from build123d import *

# Parameters (mm, degrees)
SKETCH1_W           = 29.3
SKETCH1_H           = 17
SKETCH1_R           = 1.25
BOSS_EXTRUDE1_DEPTH = 1.15
FILLET1_R           = 2.5
SKETCH2_W           = 6.962283529
SKETCH2_H           = 3.729158124
BOSS_EXTRUDE2_DEPTH = 3.5
SKETCH3_W           = 0.499386372
SKETCH3_H           = 0.1
SKETCH3_W_2         = 0.535571303
SKETCH3_W_3         = 0.69846846
CUT_EXTRUDE1_DEPTH  = 5.5
SKETCH4_W           = 6.01860052
SKETCH4_H           = 2.306780687
CUT_EXTRUDE2_DEPTH  = 3.5
SKETCH5_W           = 5.89277612
SKETCH5_H           = 4.278029639
BOSS_EXTRUDE3_DEPTH = 1
SKETCH6_W           = 3.208522229
SKETCH6_H           = 3.166580762
BOSS_EXTRUDE4_DEPTH = 1
SKETCH7_W           = 6
SKETCH7_H           = 6
BOSS_EXTRUDE5_DEPTH = 3
SKETCH8_W           = 6
SKETCH8_H           = 6
SKETCH8_R           = 1.858011724
SKETCH8_R_2         = 0.603796911
CUT_EXTRUDE3_DEPTH  = 0.5
SKETCH10_R          = 4
BOSS_EXTRUDE6_DEPTH = 10
SKETCH11_R          = 2.5
CUT_EXTRUDE4_DEPTH  = 2
SKETCH12_R          = 2.5
SKETCH12_R_2        = 2.4
CUT_EXTRUDE5_DEPTH  = 2
FILLET2_R           = 2
SKETCH13_R          = 2.5
SKETCH13_R_2        = 2.4
CUT_EXTRUDE6_DEPTH  = 2
FILLET3_R           = 2
CHAMFER1_SIZE       = 0.5
SKETCH14_R          = 3.6
SKETCH14_R_2        = 3.5
CUT_EXTRUDE7_DEPTH  = 2


with BuildPart() as part:
    # Sketch1 → Boss-Extrude1 (new body)
    with BuildSketch(Plane(origin=(0, 0, 0), x_dir=(1, 0, 0), z_dir=(0, 1, 0))):
        Rectangle(SKETCH1_W, SKETCH1_H)
        with Locations(Location((-12.15, 6, 0), (0, 0, 270))):
            Circle(SKETCH1_R, mode=Mode.SUBTRACT)
        with Locations(Location((-12.15, -6, 0), (0, 0, 270))):
            Circle(SKETCH1_R, mode=Mode.SUBTRACT)
        with Locations(Location((12.15, -6, 0), (0, 0, 270))):
            Circle(SKETCH1_R, mode=Mode.SUBTRACT)
        with Locations(Location((12.15, 6, 0), (0, 0, 270))):
            Circle(SKETCH1_R, mode=Mode.SUBTRACT)
    extrude(amount=BOSS_EXTRUDE1_DEPTH)

    # Fillet1
    fillet1_edges = [part.edges().sort_by_distance(p)[0] for p in [
        (14.65, 0.575, 8.5),
        (-14.65, 0.575, 8.5),
        (-14.65, 0.575, -8.5),
        (14.65, 0.575, -8.5),
    ]]
    fillet(fillet1_edges, radius=FILLET1_R)

    # Sketch2 → Boss-Extrude2 (add)
    with BuildSketch(Plane(origin=(0, 1.15, 0), x_dir=(1, 0, 0), z_dir=(0, 1, 0))):
        with Locations((-2.998814894, -6.635420938)):
            Rectangle(SKETCH2_W, SKETCH2_H)
    extrude(amount=BOSS_EXTRUDE2_DEPTH)

    # Sketch3 → Cut-Extrude1 (cut)
    with BuildSketch(Plane.XY.offset(8.5)):
        with Locations((-6.230263472, 1.2)):
            Rectangle(SKETCH3_W, SKETCH3_H)
        with Locations((-5.348355938, 1.2)):
            Rectangle(SKETCH3_W_2, SKETCH3_H)
        with Locations((-4.448355938, 1.2)):
            Rectangle(SKETCH3_W_2, SKETCH3_H)
        with Locations((-3.548355938, 1.2)):
            Rectangle(SKETCH3_W_2, SKETCH3_H)
        with Locations((-2.648355937, 1.2)):
            Rectangle(SKETCH3_W_2, SKETCH3_H)
        with Locations((-1.748355937, 1.2)):
            Rectangle(SKETCH3_W_2, SKETCH3_H)
        with Locations((-0.848355938, 1.2)):
            Rectangle(SKETCH3_W_2, SKETCH3_H)
        with Locations((0.133092641, 1.2)):
            Rectangle(SKETCH3_W_3, SKETCH3_H)
    extrude(amount=-CUT_EXTRUDE1_DEPTH, mode=Mode.SUBTRACT)

    # Sketch4 → Cut-Extrude2 (cut)
    with BuildSketch(Plane.XY.offset(8.5)):
        with Locations((-3.00930026, 2.964607373)):
            Rectangle(SKETCH4_W, SKETCH4_H)
    extrude(amount=-CUT_EXTRUDE2_DEPTH, mode=Mode.SUBTRACT)

    # Sketch5 → Boss-Extrude3 (add)
    with BuildSketch(Plane(origin=(0, 1.15, 0), x_dir=(1, 0, 0), z_dir=(0, 1, 0))):
        with Locations((1.792997716, 2.736680725)):
            Rectangle(SKETCH5_W, SKETCH5_H)
    extrude(amount=BOSS_EXTRUDE3_DEPTH)

    # Sketch6 → Boss-Extrude4 (add)
    with BuildSketch(Plane(origin=(0, 1.15, 0), x_dir=(1, 0, 0), z_dir=(0, 1, 0))):
        with Locations((6.406559091, -4.802297976)):
            Rectangle(SKETCH6_W, SKETCH6_H)
    extrude(amount=BOSS_EXTRUDE4_DEPTH)

    # Sketch7 → Boss-Extrude5 (add)
    with BuildSketch(Plane.XZ):
        with Locations((0, 5.5)):
            Rectangle(SKETCH7_W, SKETCH7_H)
    extrude(amount=BOSS_EXTRUDE5_DEPTH)

    # Sketch8 → Cut-Extrude3 (cut)
    # profile 1 of 2: a face of its own
    with BuildSketch(Plane.XZ.offset(3)):
        with Locations((0, 5.5)):
            Rectangle(SKETCH8_W, SKETCH8_H)
        with Locations(Location((0, 5.56772975, 0), (0, 0, 270))):
            Circle(SKETCH8_R, mode=Mode.SUBTRACT)
    # profile 2 of 2: a face of its own
    with BuildSketch(Plane.XZ.offset(3)):
        with Locations(Location((0, 5.56772975, 0), (0, 0, 270))):
            Circle(SKETCH8_R_2)
    extrude(amount=-CUT_EXTRUDE3_DEPTH, mode=Mode.SUBTRACT)

    # Sketch10 → Boss-Extrude6 (add)
    with BuildSketch(Plane.XZ):
        with Locations(Location((5, -3.5, 0), (0, 0, 90))):
            Circle(SKETCH10_R)
        with Locations(Location((-5, -3.5, 0), (0, 0, 90))):
            Circle(SKETCH10_R)
    extrude(amount=BOSS_EXTRUDE6_DEPTH)

    # Sketch11 → Cut-Extrude4 (cut)
    with BuildSketch(Plane.XZ.offset(10)):
        with Locations(Location((-5, -3.5, 0), (0, 0, 270))):
            Circle(SKETCH11_R)
        with Locations(Location((5, -3.5, 0), (0, 0, 270))):
            Circle(SKETCH11_R)
    extrude(amount=-CUT_EXTRUDE4_DEPTH, mode=Mode.SUBTRACT)

    # Sketch12 → Cut-Extrude5 (cut)
    with BuildSketch(Plane.XZ.offset(8)):
        with Locations(Location((-5, -3.5, 0), (0, 0, 270))):
            Circle(SKETCH12_R)
        with Locations(Location((-5, -3.5, 0), (0, 0, 270))):
            Circle(SKETCH12_R_2, mode=Mode.SUBTRACT)
    extrude(amount=-CUT_EXTRUDE5_DEPTH, mode=Mode.SUBTRACT)

    # Fillet2
    fillet2_edges = [part.edges().sort_by_distance(p)[0] for p in [
        (-5, -8, -1.1),
    ]]
    fillet(fillet2_edges, radius=FILLET2_R - 0.0001)  # a hair under: the kernel refuses the full size

    # Sketch13 → Cut-Extrude6 (cut)
    with BuildSketch(Plane.XZ.offset(8)):
        with Locations(Location((5, -3.5, 0), (0, 0, 270))):
            Circle(SKETCH13_R)
        with Locations(Location((5, -3.5, 0), (0, 0, 270))):
            Circle(SKETCH13_R_2, mode=Mode.SUBTRACT)
    extrude(amount=-CUT_EXTRUDE6_DEPTH, mode=Mode.SUBTRACT)

    # Fillet3
    fillet3_edges = [part.edges().sort_by_distance(p)[0] for p in [
        (5, -8, -1.1),
    ]]
    fillet(fillet3_edges, radius=FILLET3_R - 0.0001)  # a hair under: the kernel refuses the full size

    # Chamfer1
    chamfer1_edges = [part.edges().sort_by_distance(p)[0] for p in [
        (5, 0, -7.5),
        (-5, 0, -7.5),
    ]]
    chamfer(chamfer1_edges, length=CHAMFER1_SIZE)

    # Sketch14 → Cut-Extrude7 (cut)
    # profile 1 of 2: a face of its own
    with BuildSketch(Plane.XZ.offset(10)):
        with Locations(Location((-5, -3.5, 0), (0, 0, 270))):
            Circle(SKETCH14_R)
        with Locations(Location((-5, -3.5, 0), (0, 0, 270))):
            Circle(SKETCH14_R_2, mode=Mode.SUBTRACT)
    # profile 2 of 2: a face of its own
    with BuildSketch(Plane.XZ.offset(10)):
        with Locations(Location((5, -3.5, 0), (0, 0, 270))):
            Circle(SKETCH14_R)
        with Locations(Location((5, -3.5, 0), (0, 0, 270))):
            Circle(SKETCH14_R_2, mode=Mode.SUBTRACT)
    extrude(amount=-CUT_EXTRUDE7_DEPTH, mode=Mode.SUBTRACT)


solid = part.part
Input: part model. Units: mm. Frame: model coordinates. A direction names the side the tool comes from. Give positions to 0.01 mm unless a question says otherwise; leave off trailing zeros. Order: outer loops, then holes, each group sorted by start corner. A loop starts at its lowest first (then second) coordinate and runs counter-clockwise, first axis right, second up.
Q1. Section D-D on y = -7. State how many separate pieces and enclosed holes the cut face has, and give its area (3 significant figures).
Checked values:
separate pieces: 4
enclosed holes: 2
area: 89.8 mm2
Q2. Set-up query: faces 1 (the flat face through (8.011, 2, 5)), 2 (the flat face through (0, 3, 7)), 3 (the cylindrical face through (-4.249, -8.028, -5.885)). Return all of +Z, -Z, +X, -X, +Y, -Y with unobstructed straight access to the full face (end or side cutting, diameter ignored); none if empty.
Checked values:
face 1: +Z, -Z, +X, +Y
face 2: +Z
face 3: -Y
Q3. Contact query for flat-ended pins moving along their axis: pin 1 Ø4 at (x, z) = (5, -3.5) entering from -Y; pin 2 Ø1.2 at (y, z) = (-1, 6.5) entering from -X; pin 3 Ø3 at (x, z) = (12.15, -6) entering from -Y. Output: stop coordinate, or through.
Checked values:
pin 1: stops at y = -8
pin 2: stops at x = -3
pin 3: stops at y = 0
Q4. Section A-A on y = -8.5. Output: boundary loops of the cut face in (x, z), and give its area (3 significant figures).
Checked values:
outline: circle Ø8 at (-5, -3.5); circle Ø7 at (-5, -3.5); circle Ø8 at (5, -3.5); circle Ø7 at (5, -3.5); hole circle Ø7.2 at (-5, -3.5); hole circle Ø5 at (-5, -3.5); hole circle Ø7.2 at (5, -3.5); hole circle Ø5 at (5, -3.5)
area: 56.8 mm2
Q5. Ray query, probe 1 along X at (y, z) = (2, 6.5); probe 2 along X at (y, z) = (0.75, 7); probe 3 along Y at (x, z) = (-11.25, -2.25). Return the intervals inside material, ascending.
Checked values:
probe 1: x = -6.48 to -6.02, 0 to 0.48
probe 2: x = -14.44 to -12.9, -11.4 to 11.4, 12.9 to 14.44
probe 3: y = 0 to 1.15
Q6. Draft query along Z for faces 4 (the cylindrical face through (-13.37, 0.57, 5.73)), 5 (the flat face through (0, -1, 2.5)), 6 (the flat face through (0, -3, 4.8)). Return one class per face: +Z half, -Z half, draft (parallel to the pull), parting line (faces both ways), or undercut.
Checked values:
face 4: undercut
face 5: undercut
face 6: draft
Q7. Section C-C on y = -4.75. Output: boundary loops of the cut face in (x, z).
Checked values:
outline: circle Ø8 at (-5, -3.5); circle Ø8 at (5, -3.5)
Q8. Section B-B on y = -1.75. Output: boundary loops of the cut face in (x, z), and give its area (3 significant figures).
Checked values:
outline: circle Ø8 at (-5, -3.5); (-3, 2.5) - (3, 2.5) - (3, 8.5) - (-3, 8.5) - close; circle Ø8 at (5, -3.5)
area: 137 mm2
